```python
from build123d import *

# Parameters (mm, degrees)
SKETCH1_W           = 6.35
SKETCH1_H           = 60
BOSS_EXTRUDE1_DEPTH = 101.6
SKETCH2_R           = 3
CUT_EXTRUDE1_DEPTH  = 10
FILLET1_R           = 5


with BuildPart() as part:
    # Sketch1 → Boss-Extrude1 (new body)
    with BuildSketch(Plane.XY):
        with Locations((83.183251365, 0)):
            Rectangle(SKETCH1_W, SKETCH1_H)
    extrude(amount=BOSS_EXTRUDE1_DEPTH)

    # Sketch2 → Cut-Extrude1 (cut)
    with BuildSketch(Plane(origin=(86.358251365, 0, 0), x_dir=(0, 0, -1), z_dir=(1, 0, 0))):
        with Locations((-10, -20)):
            Circle(SKETCH2_R)
        with Locations((-10, 20)):
            Circle(SKETCH2_R)
        with Locations((-10, 0)):
            Circle(SKETCH2_R)
        with Locations((-50.8, 20)):
            Circle(SKETCH2_R)
        with Locations((-50.8, 0)):
            Circle(SKETCH2_R)
        with Locations((-50.8, -20)):
            Circle(SKETCH2_R)
        with Locations((-91.6, -20)):
            Circle(SKETCH2_R)
        with Locations((-91.6, 0)):
            Circle(SKETCH2_R)
        with Locations((-91.6, 20)):
            Circle(SKETCH2_R)
    extrude(amount=-CUT_EXTRUDE1_DEPTH, mode=Mode.SUBTRACT)

    # Fillet1
    fillet1_edges = [part.edges().sort_by_distance(p)[0] for p in [
        (83.183251365, 30, 101.6),
        (83.183251365, 30, 0),
        (83.183251365, -30, 0),
        (83.183251365, -30, 101.6),
    ]]
    fillet(fillet1_edges, radius=FILLET1_R)


solid = part.part
```
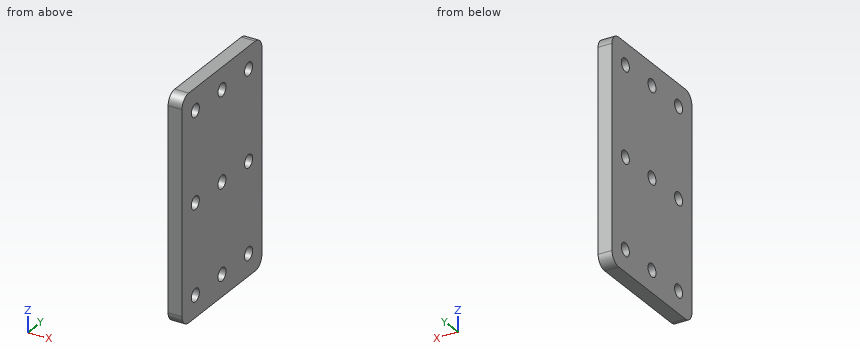
Input: part model. Units: mm. Frame: model coordinates. Coordinates: 2 decimals unless noted, no trailing zeros. Write each loop counter-clockwise with the first axis right and the second up, starting at its lowest first coordinate (ties: lowest second). Pieces come first, ordered by that corner, then holes. Notation, with made-up numbers: M 87.25,-4.5 L 128.25,-4.5 A8 ccw 128.25,9.5 Z; hole C 34.25,-36.75 d8. An arc over 180 degrees is marked long. Use one line per item in the form item = value.
Q1. First-contact query: pin 1 (8 mm diameter, centred on y = -20, z = 50.8, fed in from -X). Flat tip, straight axial feed; report the tip coordinate or a pass-through.
Answer below:
pin_1 = 80.01
Q2. Section A-A (z = 50.8). Return loops of the section in (x, y).
Answer below:
outline = M 80.01,-30 L 86.36,-30 L 86.36,-23 L 80.01,-23 Z; M 80.01,-17 L 86.36,-17 L 86.36,-3 L 80.01,-3 Z; M 80.01,3 L 86.36,3 L 86.36,17 L 80.01,17 Z; M 80.01,23 L 86.36,23 L 86.36,30 L 80.01,30 Z
Q3. Material intervals for probe 1 along Y at (x, z) = (82, 91.6); probe 2 along Y at (x, z) = (83, 92.5); probe 3 along Z at (x, y) = (83, 18), sorted ascending. Write a range as from..to.
Answer below:
probe_1 = -30..-23, -17..-3, 3..17, 23..30
probe_2 = -30..-22.86, -17.14..-2.86, 2.86..17.14, 22.86..30
probe_3 = 0..7.76, 12.24..48.56, 53.04..89.36, 93.84..101.6
Q4. Section B-B (y = 20). Return loops of the section in (x, z), plus the area to 3 significant figures.
Answer below:
outline = M 80.01,0 L 86.36,0 L 86.36,7 L 80.01,7 Z; M 80.01,13 L 86.36,13 L 86.36,47.8 L 80.01,47.8 Z; M 80.01,53.8 L 86.36,53.8 L 86.36,88.6 L 80.01,88.6 Z; M 80.01,94.6 L 86.36,94.6 L 86.36,101.6 L 80.01,101.6 Z
area = 531 mm²
Q5. Section C-C (x = 81.75). Count the separate pieces of the cut face and the enclosed holes in it, plus the area to 3 significant figures.
Answer below:
separate_pieces = 1
enclosed_holes = 9
area = 5,820 mm²
